```python
from build123d import *

# Parameters (mm, degrees)
F1_DEPTH    = 20
F0_R        = 1.25
F0_W        = 23
F0_H        = 12
F2_DEPTH    = 5
F3_R        = 1.25
F4_DEPTH    = 5
F5_T1_DEPTH = 20
F5_T3_DEPTH = 20
F5_T5_DEPTH = 35


# Not quite as in the source:
# - a fillet or chamfer that OpenCascade refuses, or shapes differently, is made with other operations: its cross-section is extruded or revolved along the edge and cut away or added


with BuildPart() as f1:
    # F0 (on Top) → F1 (new body)
    with BuildSketch(Plane.XY):
        Polygon((-10, 15), (-10, 10), (10, 10), (10, 15), (0, 15), align=None)
    extrude(amount=F1_DEPTH)

    # F0 (on Top) → F2 (join)
    with BuildSketch(Plane.XY):
        Polygon((-10, 10), (-20, 10), (-20, -10), (20, -10), (20, 10), (10, 10), align=None)
        with Locations((-13.97, 0)):
            Circle(F0_R, mode=Mode.SUBTRACT)
        Rectangle(F0_W, F0_H, mode=Mode.SUBTRACT)
        with Locations((13.97, 0)):
            Circle(F0_R, mode=Mode.SUBTRACT)
    extrude(amount=F2_DEPTH)

    # F3 (on face) → F4 (cut)
    with BuildSketch(Plane(origin=(0, 15, 0), x_dir=(-1, 0, 0), z_dir=(0, 1, 0))):
        with Locations((3.865, 17.1576076342)):
            Circle(F3_R)
        with Locations((-3.865, 17.1576076342)):
            Circle(F3_R)
    extrude(amount=-F4_DEPTH, mode=Mode.SUBTRACT)

    # F5: fillet of radius 3 on 8 edges, made by hand

    # F5_s2 → F5_t1 (join)
    with BuildSketch(Plane.YZ.offset(-10)):
        with BuildLine():
            ThreePointArc((10, 8), (9.1213203436, 5.8786796564), (7, 5))
            Line((7, 5), (10, 5))
            Line((10, 5), (10, 8))
        make_face()
    extrude(amount=F5_T1_DEPTH)

    # F5_s4 → F5_t3 (cut)
    with BuildSketch(Plane.XY.offset(-7.5)):
        with BuildLine():
            ThreePointArc((-17, 10), (-19.1213203436, 9.1213203436), (-20, 7))
            Line((-20, 7), (-20, 10))
            Line((-20, 10), (-17, 10))
        make_face()
        with BuildLine():
            ThreePointArc((20, 7), (19.1213203436, 9.1213203436), (17, 10))
            Line((17, 10), (20, 10))
            Line((20, 10), (20, 7))
        make_face()
        with BuildLine():
            ThreePointArc((17, -10), (19.1213203436, -9.1213203436), (20, -7))
            Line((20, -7), (20, -10))
            Line((20, -10), (17, -10))
        make_face()
        with BuildLine():
            ThreePointArc((-20, -7), (-19.1213203436, -9.1213203436), (-17, -10))
            Line((-17, -10), (-20, -10))
            Line((-20, -10), (-20, -7))
        make_face()
    extrude(amount=F5_T3_DEPTH, mode=Mode.SUBTRACT)

    # F5_s6 → F5_t5 (cut)
    with BuildSketch(Plane.YZ.offset(-17.5)):
        with BuildLine():
            ThreePointArc((15, 3), (14.1213203436, 0.8786796564), (12, 0))
            Line((12, 0), (15, 0))
            Line((15, 0), (15, 3))
        make_face()
    extrude(amount=F5_T5_DEPTH, mode=Mode.SUBTRACT)


solid = f1.part
```
Read the model definition and answer for the solid it produces. Units are mm, in the model's axes. A direction names the side the tool comes from. Give positions to 0.01 mm unless a question says otherwise; leave off trailing zeros. Loops run counter-clockwise (first coordinate to the right, second up) from the corner with the lowest first, then second, coordinate; pieces in that order, holes last.
Item 1: The mould has two halves that part along Y. Classify faces 1 (the flat face through (0, -6, 2)), 2 (the cylindrical face through (-19.1, 9.14, 2.46)), 3 (the flat face through (-11.5, 0, 2)), 4 (the flat face through (20, 0, 2)): released by +Y, released by -Y, zero draft, split by the parting line, or undercut.
Item 2: Find the intervals of material crossed by line 1 along Y through (x, z) = (13.97, 2.8); line 2 along Z through (x, y) = (13.5, -5.75); line 3 along Y through (x, z) = (-17, 1.75), in increasing order.
Item 3: The part is cut by section A-A (x = -9). Write down the section's boundary in (y, z), and give its area (3 significant figures).
Item 4: Each of these flat-tipped pins is pushed along its axis until it touches: pin 1 Ø8 at (x, y) = (0, -7.5) entering from -Z; pin 2 Ø6.5 at (y, z) = (9.5, 8) entering from -X; pin 3 Ø3 at (x, y) = (7, -5.5) entering from +Z; pin 4 Ø4 at (x, y) = (-6.5, 7) entering from +Z. Where does it stop, or does it pass through?
Item 5: For faces 5 (the flat face through (14, 10, 2)), 6 (the cylindrical face through (4.14, 12.54, 15.94)), 7 (the flat face through (0, 10, 14)), 8 (the flat face through (-13, 10, 2)), determine the directions among +Z, -Z, +X, -X, +Y, -Y from which every point of the face is accessible in a straight line to the end or side of a thin tool.
Item 6: The part is cut by section C-C (y = 0). Write down the section's boundary in (x, z), and give its area (3 significant figures).
Item 7: The part is cut by section B-B (y = 4). Write down the section's boundary in (x, z), and give its area (3 significant figures).
Item 8: The part is cut by section D-D (x = -4.5). Write down the section's boundary in (y, z), and give its area (3 significant figures).
Taken from the geometry:
1. face 1: undercut
1. face 2: released by +Y
1. face 3: undercut
1. face 4: zero draft
2. line 1: y = -10 to -1.25, 1.25 to 10
2. line 2: z = 0 to 5
2. line 3: y = -10 to 10
3. outline: (-10, 0) - (-6, 0) - (-6, 5) - (-10, 5) - close; (6, 0) - (12, 0) arc R3 ccw to (15, 3) - (15, 20) - (10, 20) - (10, 8) arc R3 cw to (7, 5) - (6, 5) - close
3. area: 140 mm2
4. pin 1: stops at z = 0
4. pin 2: stops at x = -19.73
4. pin 3: stops at z = 5
4. pin 4: stops at z = 5.76
5. face 5: +Z, -Z, +X, +Y
5. face 6: +Y, -Y
5. face 7: +Z, +X, -X, -Y
5. face 8: +Z, -Z, -X, +Y
6. outline: (-20, 0) - (-15.22, 0) - (-15.22, 5) - (-20, 5) - close; (-12.72, 0) - (-11.5, 0) - (-11.5, 5) - (-12.72, 5) - close; (11.5, 0) - (12.72, 0) - (12.72, 5) - (11.5, 5) - close; (15.22, 0) - (20, 0) - (20, 5) - (15.22, 5) - close
6. area: 60.0 mm2
7. outline: (-20, 0) - (-11.5, 0) - (-11.5, 5) - (-20, 5) - close; (11.5, 0) - (20, 0) - (20, 5) - (11.5, 5) - close
7. area: 85.0 mm2
8. outline: (-10, 0) - (-6, 0) - (-6, 5) - (-10, 5) - close; (6, 0) - (12, 0) arc R3 ccw to (15, 3) - (15, 16.08) - (10, 16.08) - (10, 8) arc R3 cw to (7, 5) - (6, 5) - close; (10, 18.23) - (15, 18.23) - (15, 20) - (10, 20) - close
8. area: 129 mm2
